For this review, take the finished solid that the model builds, in its own axes (mm). A direction names the side the tool comes from. Coordinates: 2 decimals unless noted, no trailing zeros. Loops run counter-clockwise (first coordinate to the right, second up) from the corner with the lowest first, then second, coordinate; pieces in that order, holes last. Notation, with made-up numbers: (-1, -5.5) -> (58, -5.5) arc R36 ccw to (58, 32.5) -> close; hole circle Ø10 at (47.5, -18). An arc over 180 degrees is marked (long way). One line per item, written item: value.
from build123d import *

# Parameters (mm, degrees)
F0_R     = 6.35
F1_DEPTH = 25.4
F2_T     = -2.54


with BuildPart() as f1:
    # F0 (on Right) → F1 (new body, symmetric)
    with BuildSketch(Plane.YZ):
        Polygon((-183.3137847563, -341.5853113772), (223.0862152437, -341.5853113772), (223.0862152437, -290.7853113772), (-162.2717357877, -290.7853113772), (-456.3637847563, 3.3067375913), (-456.3637847563, 287.0646886228), (-507.1637847563, 287.0646886228), (-507.1637847563, -17.7353113772), align=None)
        with Locations((121.4862152437, -316.9367909431)):
            Circle(F0_R, mode=Mode.SUBTRACT)
    extrude(amount=F1_DEPTH, both=True)

    # F2
    f2_openings = [f1.faces().sort_by_distance(p)[0] for p in [
        (0, 223.086215, -316.185311),
        (0, -481.763785, 287.064689),
    ]]
    offset(amount=F2_T, openings=f2_openings, kind=Kind.INTERSECTION)


solid = f1.part
1. For faces 5 (the flat face through (0, -458.904, 143)), 6 (the flat face through (0, 33, -290.785)), 7 (the flat face through (0.32, -345.699, -175.608)), 8 (the flat face through (0, 18, -339.045)), 9 (the flat face through (25.4, -306, -165)), list the 3-axis set-ups (+Z, -Z, +X, -X, +Y, -Y) from which the entire face can be reached by the end or side of a thin tool; tool diameter is ignored.
Return value:
face 5: +Z
face 6: +Z, +X, -X, +Y
face 7: none
face 8: +Y
face 9: +Z, -Z, +X, +Y, -Y
2. To check wall thickness, follow probe 1 along Y at (x, z) = (-5, 173); probe 2 along Z at (x, y) = (7, -57); probe 3 along Z at (x, y) = (-5.5, -411). State the ranges of each line that lie inside material, in increasing order. Write a range as from..to.
Return value:
probe 1: y = -507.16..-504.62, -458.9..-456.36
probe 2: z = -341.59..-339.05, -293.33..-290.79
probe 3: z = -113.9..-110.31, -45.65..-42.06
3. Take a section at B-B, the plane x = -8. Give the boundary of the cut face in (y, z), and give its area (3 significant figures).
Return value:
outline: (-507.16, -17.74) -> (-183.31, -341.59) -> (223.09, -341.59) -> (223.09, -339.05) -> (-182.26, -339.05) -> (-504.62, -16.68) -> (-504.62, 287.06) -> (-507.16, 287.06) -> close; (-458.9, 2.25) -> (-163.32, -293.33) -> (223.09, -293.33) -> (223.09, -290.79) -> (-162.27, -290.79) -> (-456.36, 3.31) -> (-456.36, 287.06) -> (-458.9, 287.06) -> close; circle Ø17.78 at (121.49, -316.94); hole circle Ø12.7 at (121.49, -316.94)
area: 5,850 mm2
4. Take a section at A-A, the plane z = 34.5. Give the boundary of the cut face in (x, y), and give its area (3 significant figures).
Return value:
outline: (-25.4, -507.16) -> (25.4, -507.16) -> (25.4, -456.36) -> (-25.4, -456.36) -> close; hole (-22.86, -504.62) -> (22.86, -504.62) -> (22.86, -458.9) -> (-22.86, -458.9) -> close
area: 490 mm2
5. Take a section at C-C, the plane y = 20. Give the boundary of the cut face in (x, z), and give its area (3 significant figures).
Return value:
outline: (-25.4, -341.59) -> (25.4, -341.59) -> (25.4, -290.79) -> (-25.4, -290.79) -> close; hole (-22.86, -339.05) -> (22.86, -339.05) -> (22.86, -293.33) -> (-22.86, -293.33) -> close
area: 490 mm2
6. The part is to be moulded in two halves that separate along Y. For faces 1 (the flat face through (-24, 223.086, -318)), 2 (the flat face through (-24, -480, 287.065)), 3 (the flat face through (-22.86, -304, -164)), 4 (the flat face through (0.32, -309.045, -147.604)), say which applies: pulls with the +Y half, pulls with the -Y half, needs draft (parallel to the pull), parting line crosses it, or undercut.
Return value:
face 1: pulls with the +Y half
face 2: needs draft
face 3: undercut
face 4: undercut
7. Insertion check: pin 1 Ø1.5 at (x, y) = (8.5, -305) entering from +Z; pin 2 Ø12 at (x, y) = (14.5, -116) entering from +Z; pin 3 Ø10 at (x, y) = (-20, -269.5) entering from +Z; pin 4 Ø16.5 at (y, z) = (121.49, -316.94) entering from +X. Each pin has a flat end and moves straight along its axis. Give the tip position at first contact, or say it passes through.
Return value:
pin 1: stops at z = -147.31
pin 2: stops at z = -290.79
pin 3: stops at z = -178.56
pin 4: stops at x = 25.4
